Build history of the part. All positions in model axes, mm. A direction names the side the tool comes from. Round coordinates to 2 decimals unless told otherwise and drop trailing zeros. Loops run counter-clockwise (first coordinate to the right, second up) from the corner with the lowest first, then second, coordinate; pieces in that order, holes last. Notation, with made-up numbers: (-31, 85.5) - (22, 85.5) arc R16 ccw to (22, 110.5) - close; hole circle Ø3 at (64, -28.75). An arc over 180 degrees is marked (long way). Answer as CSV lines item,"result". Start each with the question number.
```python
from build123d import *

# Parameters (mm, degrees)
ESQUISSE1_W             = 43.6
ESQUISSE1_H             = 130
BOSS_EXTRU_1_DEPTH      = 6
ENL_V_MAT_EXTRU_1_DEPTH = 6
ESQUISSE4_W             = 15.6
ESQUISSE4_H             = 6
BOSS_EXTRU_2_DEPTH      = 6
ESQUISSE6_W             = 10
ESQUISSE6_H             = 6
ESQUISSE6_W_2           = 5
ESQUISSE6_H_2           = 6.5
ENL_V_MAT_EXTRU_3_DEPTH = 6
CONG_8_R                = 2
CONG_9_R                = 2
ESQUISSE7_R             = 1.5
ENL_V_MAT_EXTRU_4_DEPTH = 6


with BuildPart() as part:
    # Esquisse1 → Boss.-Extru.1 (new body)
    with BuildSketch(Plane.XY):
        with Locations((21.8, 65)):
            Rectangle(ESQUISSE1_W, ESQUISSE1_H)
    extrude(amount=BOSS_EXTRU_1_DEPTH)

    # Esquisse2 → Enlèv. mat.-Extru.1 (cut)
    with BuildSketch(Plane.XY.offset(6)):
        Polygon((43.6, 0), (33.3, 0), (33.3, 120), (43.6, 125), align=None)
        Polygon((10.3, 120), (0, 125), (0, 0), (10.3, 0), align=None)
    extrude(amount=-ENL_V_MAT_EXTRU_1_DEPTH, mode=Mode.SUBTRACT)

    # Esquisse4 → Boss.-Extru.2 (add)
    with BuildSketch(Plane.XY.offset(6)):
        with Locations((21.8, 133)):
            Rectangle(ESQUISSE4_W, ESQUISSE4_H)
    extrude(amount=-BOSS_EXTRU_2_DEPTH)

    # Esquisse6 → Enlèv. mat.-Extru.3 (cut)
    with BuildSketch(Plane.XY.offset(6)):
        with Locations((15.3, 9)):
            Rectangle(ESQUISSE6_W, ESQUISSE6_H)
        with Locations((12.8, 113.75)):
            Rectangle(ESQUISSE6_W_2, ESQUISSE6_H_2)
    extrude(amount=-ENL_V_MAT_EXTRU_3_DEPTH, mode=Mode.SUBTRACT)

    # Congé8
    cong_8_edges = [part.edges().sort_by_distance(p)[0] for p in [
        (33.3, 0, 3),
        (10.3, 0, 3),
    ]]
    fillet(cong_8_edges, radius=CONG_8_R)

    # Congé9
    cong_9_edges = [part.edges().sort_by_distance(p)[0] for p in [
        (43.6, 125, 3),
        (0, 125, 3),
    ]]
    fillet(cong_9_edges, radius=CONG_9_R)

    # Esquisse7 → Enlèv. mat.-Extru.4 (cut)
    with BuildSketch(Plane.XY.offset(6)):
        with Locations((28.3, 3)):
            Circle(ESQUISSE7_R)
    extrude(amount=-ENL_V_MAT_EXTRU_4_DEPTH, mode=Mode.SUBTRACT)


solid = part.part
```
Q1. Pin check, flat tips, straight feed: pin 1 Ø3 at (y, z) = (47, 3.5) entering from -X; pin 2 Ø1 at (x, y) = (21, 88) entering from -Z; pin 3 Ø1.8 at (y, z) = (132.5, 2) entering from -X; pin 4 Ø1.8 at (y, z) = (134, 4) entering from +X. Stop position of each tip, or through.
Q2. Two-plate mould, pull along X, no slides. Class faces 4 (the flat face through (0, 128, 3)), 5 (the cylindrical face through (29.686, 2.425, 3.042)), 6 (the flat face through (33.3, 60, 3)): released by +X, released by -X, zero draft, split by the parting line, or undercut.
Q3. Band-saw the part on A-A, the plane z = 4.7. List the corners of the cut face in (x, y).
Q4. Band-saw the part on D-D, the plane y = 114.5. List the corners of the cut face in (x, z).
Q5. Tool access for faces 1 (the flat face through (10.3, 4, 3)), 2 (the flat face through (13, 110.5, 3)), 3 (the flat face through (29.6, 133, 3)): list every direction of +Z, -Z, +X, -X, +Y, -Y with a clear straight run to the whole face (end or side of a thin tool).
Q6. Wall check: probe 1 along Y at (x, z) = (12, 2.25); probe 2 along Y at (x, z) = (28.3, 4.6); probe 3 along Y at (x, z) = (19, 1.5). Give the ranges that are in metal, low to high. Write a range as [from, to].
Q7. Band-saw the part on B-B, the plane x = 28.3. List the corners of the cut face in (y, z).
Q8. Band-saw the part on C-C, the plane y = 68.5. List the corners of the cut face in (x, z).
Reported:
1,pin 1,"stops at x = 10.3"
1,pin 2,"stops at z = 0"
1,pin 3,"stops at x = 14"
1,pin 4,"stops at x = 29.6"
2,face 4,"released by -X"
2,face 5,"undercut"
2,face 6,"released by +X"
3,outline,"(0, 126.25) arc R2 ccw to (1.13, 124.45) - (10.3, 120) - (10.3, 117) - (15.3, 117) - (15.3, 110.5) - (10.3, 110.5) - (10.3, 12) - (20.3, 12) - (20.3, 6) - (10.3, 6) - (10.3, 2) arc R2 ccw to (12.3, 0) - (31.3, 0) arc R2 ccw to (33.3, 2) - (33.3, 120) - (42.47, 124.45) arc R2 ccw to (43.6, 126.25) - (43.6, 130) - (29.6, 130) - (29.6, 136) - (14, 136) - (14, 130) - (0, 130) - close; hole circle Ø3 at (28.3, 3)"
4,outline,"(15.3, 0) - (33.3, 0) - (33.3, 6) - (15.3, 6) - close"
5,face 1,"+Z, -Z, -X, -Y"
5,face 2,"+Z, -Z, -X"
5,face 3,"+Z, -Z, +X, +Y"
6,probe 1,"y = [0.02, 6], [12, 110.5], [117, 130]"
6,probe 2,"y = [0, 1.5], [4.5, 136]"
6,probe 3,"y = [0, 6], [12, 136]"
7,outline,"(0, 0) - (1.5, 0) - (1.5, 6) - (0, 6) - close; (4.5, 0) - (136, 0) - (136, 6) - (4.5, 6) - close"
8,outline,"(10.3, 0) - (33.3, 0) - (33.3, 6) - (10.3, 6) - close"
